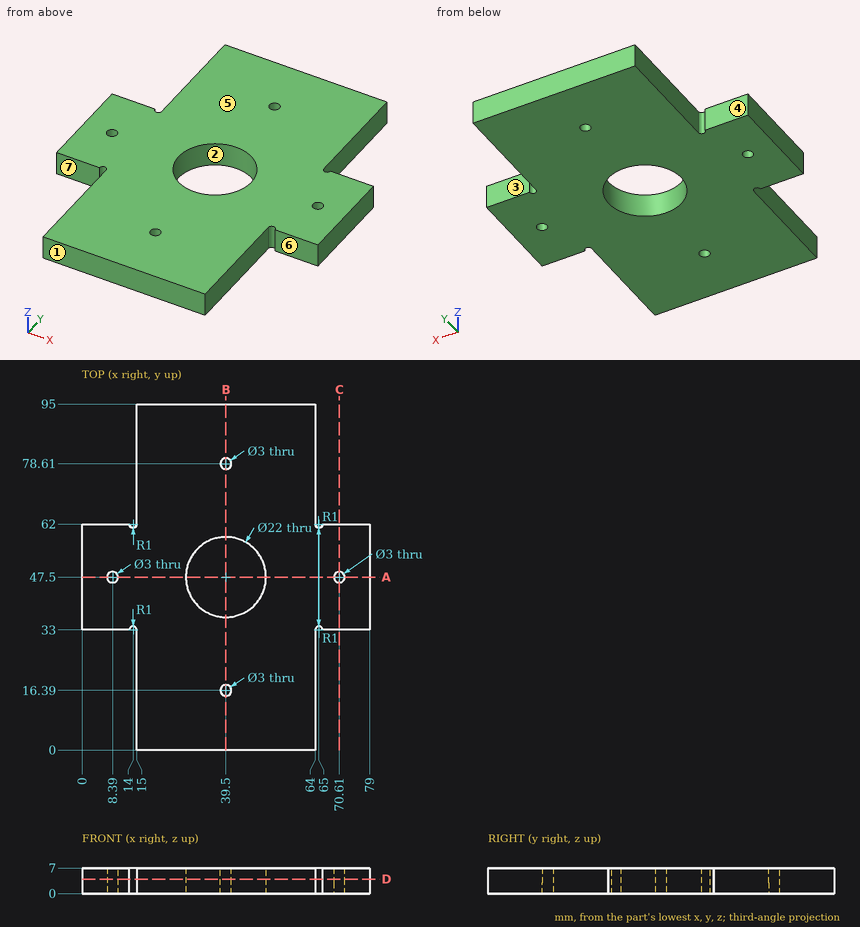
Verification items for this drawing (mm, ordinates from the low corner). A direction names the side the tool comes from. Give positions to 0.01 mm unless a question says otherwise; leave off trailing zeros. Loops run counter-clockwise (first coordinate to the right, second up) from the corner with the lowest first, then second, coordinate; pieces in that order, holes last. Notation, with made-up numbers: M 67,25 L 74,25 A11 cw 74,33 Z; hole C -2.5,28 d4. An arc over 180 degrees is marked long. Answer as a JSON object with one key per item and string values. Group by question number.
Item 1: Sectioned sample at D-D on z = 4. Record the boundary of the cut face in (x, y).
Item 2: Sectioned sample at C-C on x = 70.61. Record the boundary of the cut face in (y, z), plus the area to 3 significant figures.
Item 3: Gauge pin test, flat ends, axial feed: pin 1 (2 mm diameter, centred on x = 6.5, z = 3, fed in from -Y); pin 2 (3.5 mm diameter, centred on y = 14.5, z = 4.5, fed in from +X); pin 3 (3 mm diameter, centred on x = 64, z = 3.5, fed in from -Y). Record the tip position at first contact, or that the pin passes through.
Item 4: Access from +Z, -Z, +X, -X, +Y, -Y to the whole of each face (thin tool, end or side, straight path). Record for the marked faces 3, 4, 5, 6 and 7.
Item 5: Mould release check, pull along X, two halves, no side actions. Record for the marked faces 1 and 2: pulls with the +X half, pulls with the -X half, needs draft (parallel to the pull), parting line crosses it, or undercut.
Item 6: Material ranges on L1, parallel to Y at x = 39.5, z = 2.75; L2, parallel to X at y = 78.5, z = 2; L3, parallel to Y at x = 70.61, z = 2.25, recorded low to high.
Item 7: Sectioned sample at A-A on y = 47.5. Record the boundary of the cut face in (x, z).
Item 8: Sectioned sample at B-B on x = 39.5. Record the boundary of the cut face in (y, z).
Findings below:
{
 "1": {"outline": "M 0,33 L 13,33 A1 cw 15,33 L 15,0 L 64,0 L 64,33 A1 cw 66,33 L 79,33 L 79,62 L 66,62 A1 cw 64,62 L 64,95 L 15,95 L 15,62 A1 cw 13,62 L 0,62 Z; hole C 8.39,47.5 d3; hole C 39.5,47.5 d22; hole C 39.5,16.39 d3; hole C 39.5,78.61 d3; hole C 70.61,47.5 d3"},
 "2": {"outline": "M 33,0 L 46,0 L 46,7 L 33,7 Z; M 49,0 L 62,0 L 62,7 L 49,7 Z", "area": "182 mm2"},
 "3": {"pin 1": "y = 33", "pin 2": "x = 64", "pin 3": "y = 0"},
 "4": {"face 3": "+Z, -Z, +X, +Y", "face 4": "+Z, -Z, -X, +Y", "face 5": "+Z, +X, -X, +Y, -Y", "face 6": "+Z, -Z, +X, -Y", "face 7": "+Z, -Z, -X, -Y"},
 "5": {"face 1": "needs draft", "face 2": "undercut"},
 "6": {"L1": "0 to 14.89, 17.89 to 36.5, 58.5 to 77.11, 80.11 to 95", "L2": "15 to 38, 41 to 64", "L3": "33 to 46, 49 to 62"},
 "7": {"outline": "M 0,0 L 6.89,0 L 6.89,7 L 0,7 Z; M 9.89,0 L 28.5,0 L 28.5,7 L 9.89,7 Z; M 50.5,0 L 69.11,0 L 69.11,7 L 50.5,7 Z; M 72.11,0 L 79,0 L 79,7 L 72.11,7 Z"},
 "8": {"outline": "M 0,0 L 14.89,0 L 14.89,7 L 0,7 Z; M 17.89,0 L 36.5,0 L 36.5,7 L 17.89,7 Z; M 58.5,0 L 77.11,0 L 77.11,7 L 58.5,7 Z; M 80.11,0 L 95,0 L 95,7 L 80.11,7 Z"}
}
